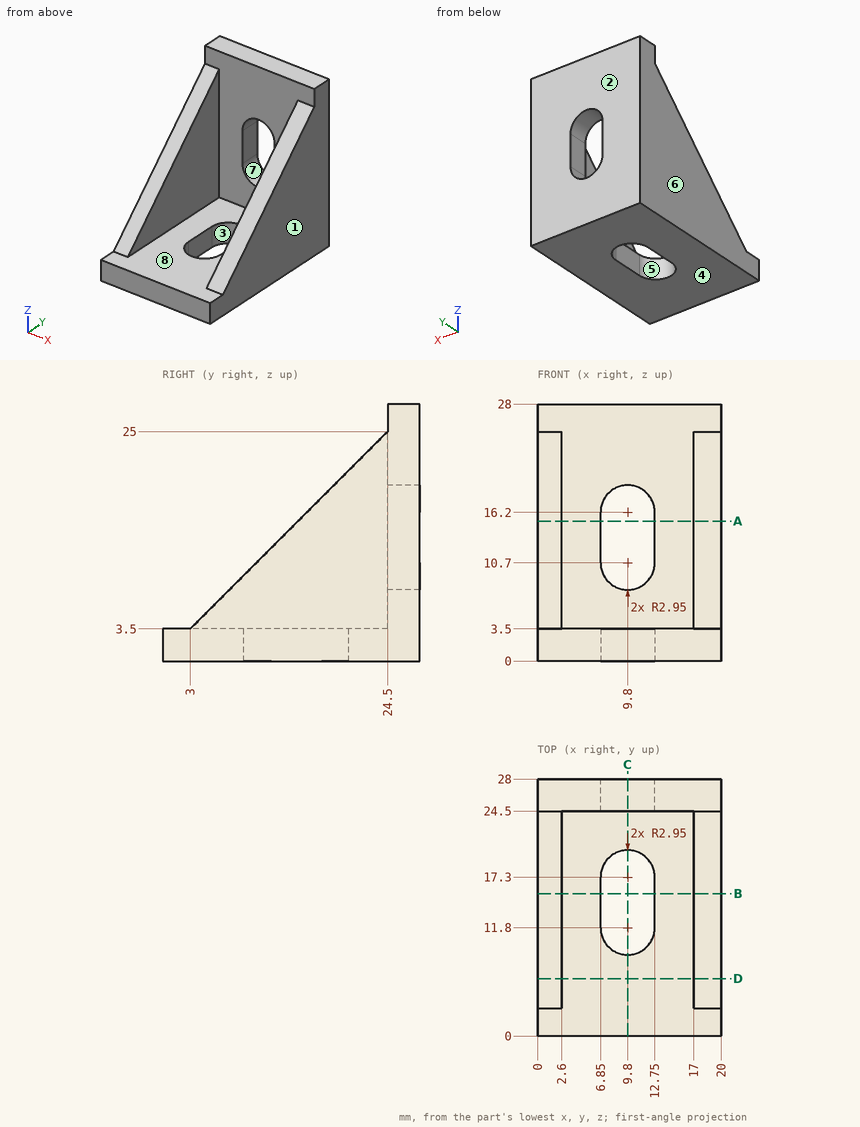
Here's the drawing with two shaded views (mm, measured from the low corner). I have some questions. A direction names the side the tool comes from. Give positions to 0.01 mm unless a question says otherwise; leave off trailing zeros. Order: outer loops, then holes, each group sorted by start corner. A loop starts at its lowest first (then second) coordinate and runs counter-clockwise, first axis right, second up.
Q1. If I drill on line 1 along X through (y, z) = (21.5, 16.75); line 2 along Z through (x, y) = (9.5, 24.25); line 3 along Y through (x, z) = (5.75, 22.5), over which ranges is the centre line in solid material (lowest first)?
Q2. I'm going to push flat-ended pins straight in: P1, Ø6.5, axis at y = 9, z = 14.5, coming from the +X side; P2, Ø4, axis at x = 18, y = 3.5, coming from the +Z side; P3, Ø10, axis at x = 11.5, y = 16.5, coming from the +Z side. Where does each tip first touch, or does it pass through?
Q3. Suppose I cut it at D-D, the plane y = 6.25. Write out the boundary of the cut face in (x, z), and give its area (3 significant figures).
Q4. Suppose I cut it at C-C, the plane x = 9.8. Write out the boundary of the cut face in (y, z).
Q5. Suppose I cut it at B-B, the plane y = 15.5. Write out the boundary of the cut face in (x, z).
Q6. We'd pull the mould along X, two halves only. Please class the marked faces 1, 2 and 3: +X half, -X half, draft (parallel to the pull), parting line (faces both ways), or undercut.
Q7. For the marked faces 4, 5, 6, 7 and 8, which set-ups out of +Z, -Z, +X, -X, +Y, -Y let a thin tool reach every point of the face, with its end or its side?
Q8. Suppose I cut it at A-A, the plane z = 15.25. Write out the boundary of the cut face in (x, y).
Solution:
1. line 1: x = 0 to 2.6, 17 to 20
1. line 2: z = 0 to 3.5
1. line 3: y = 24.5 to 28
2. P1: passes through
2. P2: stops at z = 6
2. P3: stops at z = 3.5
3. outline: (0, 0) - (20, 0) - (20, 6.75) - (17, 6.75) - (17, 3.5) - (2.6, 3.5) - (2.6, 6.75) - (0, 6.75) - close
3. area: 88.2 mm2
4. outline: (0, 0) - (8.85, 0) - (8.85, 3.5) - (0, 3.5) - close; (20.25, 0) - (28, 0) - (28, 7.75) - (24.5, 7.75) - (24.5, 3.5) - (20.25, 3.5) - close; (24.5, 19.15) - (28, 19.15) - (28, 28) - (24.5, 28) - close
5. outline: (0, 0) - (6.85, 0) - (6.85, 3.5) - (2.6, 3.5) - (2.6, 16) - (0, 16) - close; (12.75, 0) - (20, 0) - (20, 16) - (17, 16) - (17, 3.5) - (12.75, 3.5) - close
6. face 1: +X half
6. face 2: draft
6. face 3: undercut
7. face 4: -Z, +X, -X, +Y, -Y
7. face 5: +Z, -Z
7. face 6: +Z, -Z, -X, +Y, -Y
7. face 7: +Y, -Y
7. face 8: +Z, -Y
8. outline: (0, 14.75) - (2.6, 14.75) - (2.6, 24.5) - (6.85, 24.5) - (6.85, 28) - (0, 28) - close; (12.75, 24.5) - (17, 24.5) - (17, 14.75) - (20, 14.75) - (20, 28) - (12.75, 28) - close
